Read the model definition and answer for the solid it produces. Units are mm, in the model's axes. Face numbers are marked on the shaded views. Coordinates: 2 decimals unless noted, no trailing zeros. Loops run counter-clockwise (first coordinate to the right, second up) from the corner with the lowest first, then second, coordinate; pieces in that order, holes last. Notation, with made-up numbers: (-25.5, 88) -> (-19.5, 88) arc R25 cw to (-19.5, 121) -> close; hole circle Ø1 at (-10.5, -8.75). An arc over 180 degrees is marked (long way). Answer as a JSON object with one key per item and string values. Group by question number.
1) Section C-C, the plane y = 10.5 is taken. Give the vertices of the cut face in (x, z).
2) Consider probe 1 along Y at (x, z) = (-17.75, 0.4); probe 2 along Y at (x, z) = (-19, 2.75); probe 3 along X at (y, z) = (3.25, 1.55). Determine where each line is inside the solid, lowest interval first. Write a range as [from, to].
3) Section A-A, the plane z = 0.8 is taken. Give the vertices of the cut face in (x, y), plus the area to 3 significant figures.
4) Section D-D, the plane x = -8.5 is taken. Give the vertices of the cut face in (y, z), plus the area to 3 significant figures.
5) Flat-ended cylindrical pins translate along their axes: P1, Ø1, axis at y = 9.5, z = 2.5, coming from the -X side; P2, Ø1.5, axis at y = 2.5, z = 1.5, coming from the +X side. Find the tip coordinate at first contact, or state that the pin passes through.
6) Section B-B, the plane x = -17 is taken. Give the vertices of the cut face in (y, z), plus the area to 3 significant figures.
7) Determine the mould class of the marked faces 1, 2, 3 and 4 for opening direction X: released by +X, released by -X, zero draft, split by the parting line, or undercut.
from build123d import *

# Parameters (mm, degrees)
SKETCH1_R           = 1.5
BOSS_EXTRUDE1_DEPTH = 3


with BuildPart() as part:
    # Sketch1 → Boss-Extrude1 (new body)
    with BuildSketch(Plane.XY):
        with BuildLine():
            Line((-20.398188463, 8.511583185), (-16.398188463, 1.511583185))
            ThreePointArc((-16.398188463, 1.511583185), (-15.299239491, 0.405269721), (-13.793459037, 0))
            Line((-13.793459037, 0), (-10.793459037, 0))
            Line((-10.793459037, 0), (-10.793459037, 5.371708245))
            Line((-10.793459037, 5.371708245), (-6.965474487, 4.463821993))
            Line((-6.965474487, 4.463821993), (-15.811037483, 12.251667113))
            ThreePointArc((-15.811037483, 12.251667113), (-19.689210528, 12.3251078), (-20.398188463, 8.511583185))
        make_face()
        with Locations((-17.793459037, 10)):
            Circle(SKETCH1_R, mode=Mode.SUBTRACT)
        with Locations((-13.793459037, 3)):
            Circle(SKETCH1_R, mode=Mode.SUBTRACT)
    extrude(amount=BOSS_EXTRUDE1_DEPTH)


solid = part.part
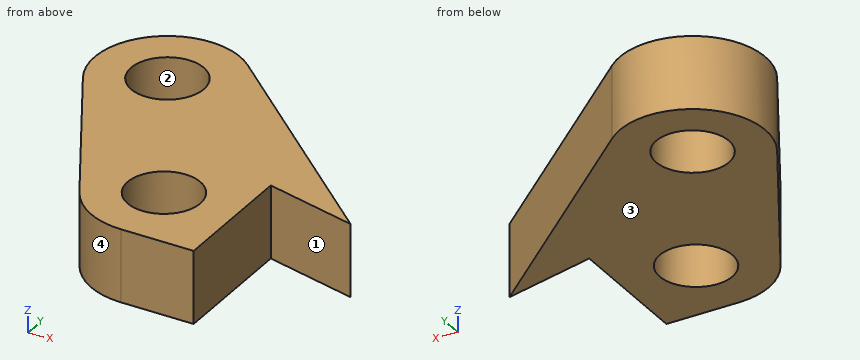
Determined:
{
 "1": {"outline": "(-20.75, 0) -> (-19.21, 0) -> (-19.21, 3) -> (-20.75, 3) -> close; (-16.38, 0) -> (-13.82, 0) -> (-13.82, 3) -> (-16.38, 3) -> close"},
 "2": {"probe 1": "[3.88, 8.5], [11.5, 13]", "probe 2": "[6.06, 9.11], [10.89, 12.75]", "probe 3": "[-17.39, -15.27], [-12.31, -10.79]"},
 "3": {"outline": "(-20.4, 8.51) -> (-16.4, 1.51) arc R3 ccw to (-13.79, 0) -> (-10.79, 0) -> (-10.79, 5.37) -> (-6.97, 4.46) -> (-15.81, 12.25) arc R3 ccw to start; hole circle Ø3 at (-17.79, 10); hole circle Ø3 at (-13.79, 3)", "area": "78.6 mm²"},
 "4": {"outline": "(4.83, 0) -> (5.81, 0) -> (5.81, 3) -> (4.83, 3) -> close", "area": "2.96 mm²"},
 "5": {"P1": "x = -20.79", "P2": "x = -10.79"},
 "6": {"outline": "(2.56, 0) -> (8.73, 0) -> (8.73, 3) -> (2.56, 3) -> close; (11.27, 0) -> (12.89, 0) -> (12.89, 3) -> (11.27, 3) -> close", "area": "23.3 mm²"},
 "7": {"face 1": "undercut", "face 2": "undercut", "face 3": "zero draft", "face 4": "released by -X"}
}
